The listing builds one solid part. Answer for the finished solid, in the listing's coordinates (mm). Face numbers are marked on the shaded views. A direction names the side the tool comes from. Round coordinates to 2 decimals unless told otherwise and drop trailing zeros. Loops run counter-clockwise (first coordinate to the right, second up) from the corner with the lowest first, then second, coordinate; pieces in that order, holes last. Notation, with made-up numbers: (75, -16.5) - (133, -16.5) arc R14 cw to (133, 1.5) - close; hole circle Ø1 at (64.25, 13.5). An arc over 180 degrees is marked (long way). Write item = value, one per line. Start each with the question number.
1) Section B-B, the plane z = 5.25 is taken. Give the number of separate pieces and of enclosed holes in the cut face, and give its area (3 significant figures).
2) Section A-A, the plane x = 0 is taken. Determine the outline of the cut face in (y, z), and give its area (3 significant figures).
3) For a pull along Y with two mould halves and no side action, classify the marked faces 4, 5 and 6 as released by +Y, released by -Y, zero draft, split by the parting line, or undercut.
4) Given pin 1 Ø4 at (x, z) = (-9, 5) entering from +Y; pin 2 Ø7 at (x, y) = (19.45, 19.45) entering from -Z; pin 3 Ø1.5 at (y, z) = (5.5, 6) entering from +X, each flat-ended and moving along its own axis, determine where each tip first touches the part or whether it passes through.
5) Section C-C, the plane y = -9 is taken. Determine the outline of the cut face in (x, z), and give its area (3 significant figures).
6) A tool of negligible diameter and unlimited length cuts with its end or side. For the marked faces 1, 2 and 3, from which of +Z, -Z, +X, -X, +Y, -Y can it reach the whole face along a straight path? Write none if from no direction.
7) Straight lines are drawn through the part: line 1 along Y through (x, z) = (27.5, 2.3); line 2 along Y through (x, z) = (27.5, 6.6); line 3 along X through (y, z) = (18, 2.75). For each, find the intervals that lie inside material, in ascending order.
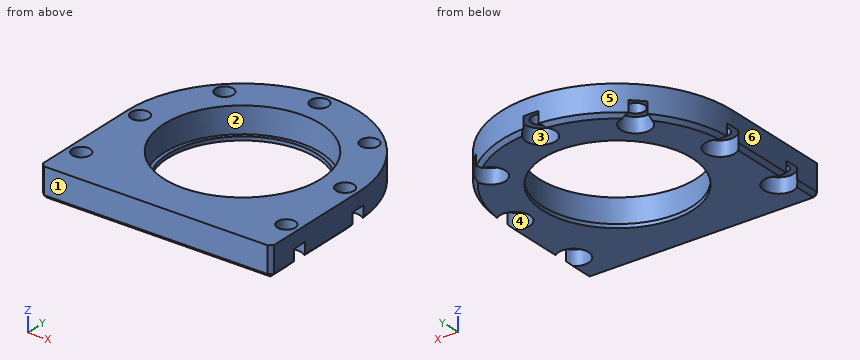
from build123d import *

# Parameters (mm, degrees)
EXTRUDE_1_DEPTH              = 8
CHAMFER_1_SIZE               = 1
HOLE_WIZARD_M4_1_D           = 4.8
HOLE_WIZARD_M4_1_CBORE_D     = 8
HOLE_WIZARD_M4_1_CBORE_DEPTH = 4
PATTERN_CIRCULAR_1_COUNT     = 8
SKETCH_11_R                  = 21
CUT_EXTRUDE_8_DEPTH          = 7
SKETCH_12_R                  = 20
CUT_EXTRUDE_9_DEPTH          = 2.0000001
HOLE_WIZARD_M4_2_D           = 4.8
HOLE_WIZARD_M4_2_CBORE_D     = 8
HOLE_WIZARD_M4_2_CBORE_DEPTH = 4


with BuildPart() as part:
    # ｽｹｯﾁ1 → ﾎﾞｽ - 押し出し1 (new body)
    with BuildSketch(Plane.XY):
        with BuildLine():
            Line((31, -31), (-31, -31))
            Line((-31, -31), (-31, 0))
            ThreePointArc((-31, 0), (0, 31), (31, 0))
            Line((31, 0), (31, -31))
        make_face()
    extrude(amount=EXTRUDE_1_DEPTH)

    # 面取り1
    chamfer_1_edges = [part.edges().sort_by_distance(p)[0] for p in [
        (31, -15.5, 0),
        (0, -31, 0),
        (-31, -15.5, 0),
        (0, 31, 0),
        (31, -31, 4),
        (-31, -31, 4),
    ]]
    chamfer(chamfer_1_edges, length=CHAMFER_1_SIZE)

    # M4 穴付きねじ用座ぐり穴1 (through all)
    with Locations(Plane(origin=(0, 0, 0), x_dir=(1, 0, 0), z_dir=(0, 0, -1))):
        with Locations((0, -27.5)):
            hole_wizard_m4_1 = CounterBoreHole(HOLE_WIZARD_M4_1_D / 2, HOLE_WIZARD_M4_1_CBORE_D / 2, HOLE_WIZARD_M4_1_CBORE_DEPTH)

    # 円形ﾊﾟﾀｰﾝ1: M4 穴付きねじ用座ぐり穴1 ×8 about axis, 3 skipped
    pattern_circular_1_axis = Axis((0, 0, 0), (0, 0, -1))
    add([hole_wizard_m4_1.rotate(pattern_circular_1_axis, i * 360 / PATTERN_CIRCULAR_1_COUNT) for i in range(1, PATTERN_CIRCULAR_1_COUNT) if i not in (3, 4, 5)], mode=Mode.SUBTRACT)

    # ｽｹｯﾁ11 → ｶｯﾄ - 押し出し8 (cut)
    with BuildSketch(Plane.XY.offset(8)):
        Circle(SKETCH_11_R)
    extrude(amount=-CUT_EXTRUDE_8_DEPTH, mode=Mode.SUBTRACT)

    # ｽｹｯﾁ12 → ｶｯﾄ - 押し出し9 (cut, through all)
    with BuildSketch(Plane.XY.offset(1)):
        Circle(SKETCH_12_R)
    extrude(amount=-CUT_EXTRUDE_9_DEPTH, mode=Mode.SUBTRACT)

    # M4 穴付きねじ用座ぐり穴2 (through all)
    with Locations(Plane(origin=(0, 0, 0), x_dir=(-1, 0, 0), z_dir=(0, 0, -1))):
        with Locations((27.5, -21), (-27.5, -21)):
            CounterBoreHole(HOLE_WIZARD_M4_2_D / 2, HOLE_WIZARD_M4_2_CBORE_D / 2, HOLE_WIZARD_M4_2_CBORE_DEPTH)


solid = part.part
Geometry check:
q1.separate_pieces = 1
q1.enclosed_holes = 8
q1.area = 1,920 mm2
q2.outline = (-31, 1) - (-30, 0) - (-20, 0) - (-20, 1) - (-21, 1) - (-21, 8) - (-31, 8) - close; (20, 0) - (23.5, 0) - (23.5, 4) - (25.1, 4) - (25.1, 8) - (21, 8) - (21, 1) - (20, 1) - close; (29.9, 4) - (31, 4) - (31, 8) - (29.9, 8) - close
q2.area = 112 mm2
q3.face_4 = undercut
q3.face_5 = released by +Y
q3.face_6 = zero draft
q4.pin_1 = 30.2
q4.pin_2 = 4
q4.pin_3 = 30.63
q5.outline = (-31, 1) - (-30, 0) - (-17.86, 0) - (-17.86, 1) - (-18.97, 1) - (-18.97, 8) - (-31, 8) - close; (17.86, 0) - (30, 0) - (31, 1) - (31, 8) - (18.97, 8) - (18.97, 1) - (17.86, 1) - close
q5.area = 194 mm2
q6.face_1 = +Z, -Z, +X, -X, -Y
q6.face_2 = +Z
q6.face_3 = -Z
q7.line_1 = -31 to -25, -17 to -4, 4 to 14.31
q7.line_2 = -31 to -23.4, -18.6 to -2.4, 2.4 to 14.31
q7.line_3 = -25.24 to -23.18, -15.72 to -10.82, 10.82 to 15.72, 23.18 to 25.24
